from build123d import *

# Parameters (mm, degrees)
P_IDAT_VYSUNUT_M1_DEPTH  = 31
SKICA3_R                 = 3.5
ODEBRAT_VYSUNUT_M1_DEPTH = 4
SKICA4_R                 = 2
ODEBRAT_VYSUNUT_M2_DEPTH = 36.80851854
SKICA5_R                 = 2
ODEBRAT_VYSUNUT_M3_DEPTH = 10


with BuildPart() as part:
    # Skica2 → Přidat vysunutím1 (new body)
    with BuildSketch(Plane.XY):
        with BuildLine():
            Line((15.5, -4.5), (15.5, 4.5))
            Line((15.5, 4.5), (-15.5, 4.5))
            Line((-15.5, 4.5), (-15.5, -4.5))
            Line((-15.5, -4.5), (-4, -4.5))
            ThreePointArc((-4, -4.5), (0, -0.5), (4, -4.5))
            Line((4, -4.5), (15.5, -4.5))
        make_face()
    extrude(amount=P_IDAT_VYSUNUT_M1_DEPTH)

    # Skica3 → Odebrat vysunutím1 (cut)
    with BuildSketch(Plane(origin=(0, 4.5, 0), x_dir=(1, 0, 0), z_dir=(0, 1, 0))):
        with Locations(Location((9.75, -5.75, 0), (0, 0, 270))):
            Circle(SKICA3_R)
        with Locations(Location((9.75, -25.25, 0), (0, 0, 90))):
            Circle(SKICA3_R)
        with Locations(Location((-9.75, -5.75, 0), (0, 0, 90))):
            Circle(SKICA3_R)
        with Locations(Location((-9.75, -25.25, 0), (0, 0, 270))):
            Circle(SKICA3_R)
    extrude(amount=-ODEBRAT_VYSUNUT_M1_DEPTH, mode=Mode.SUBTRACT)

    # Skica4 → Odebrat vysunutím2 (cut, through all)
    with BuildSketch(Plane(origin=(0, 4.5, 0), x_dir=(1, 0, 0), z_dir=(0, 1, 0))):
        with Locations(Location((9.75, -5.75, 0), (0, 0, 270))):
            Circle(SKICA4_R)
        with Locations(Location((-9.75, -5.75, 0), (0, 0, 270))):
            Circle(SKICA4_R)
        with Locations(Location((-9.75, -25.25, 0), (0, 0, 270))):
            Circle(SKICA4_R)
        with Locations(Location((9.75, -25.25, 0), (0, 0, 270))):
            Circle(SKICA4_R)
    extrude(amount=-ODEBRAT_VYSUNUT_M2_DEPTH, mode=Mode.SUBTRACT)

    # Skica5 → Odebrat vysunutím3 (cut)
    with BuildSketch(Plane(origin=(15.5, 0, 0), x_dir=(0, 0, -1), z_dir=(1, 0, 0))):
        with Locations((-15.5, 0)):
            Circle(SKICA5_R)
    extrude(amount=-ODEBRAT_VYSUNUT_M3_DEPTH, mode=Mode.SUBTRACT)


solid = part.part
Work out the finished part from the listing and answer in its coordinate system (mm). A direction names the side the tool comes from. Give positions to 0.01 mm unless a question says otherwise; leave off trailing zeros. Loops run counter-clockwise (first coordinate to the right, second up) from the corner with the lowest first, then second, coordinate; pieces in that order, holes last. Notation, with made-up numbers: (2.5, 33.5) -> (6.5, 33.5) arc R22 cw to (6.5, 49.5) -> close; hole circle Ø1 at (-29, 32). An arc over 180 degrees is marked (long way). Use a Markdown table: item, result. Add a question column.
1. Find the intervals of material crossed by probe 1 along X at (y, z) = (3.15, 25.25); probe 2 along Z at (x, y) = (-9, -0.5); probe 3 along X at (y, z) = (2.25, 3), in increasing order.
2. Section D-D on x = 14.5 is taken. Determine the outline of the cut face in (y, z).
3. Flat-ended cylindrical pins translate along their axes: pin 1 Ø3 at (y, z) = (0, 15.5) entering from +X; pin 2 Ø5 at (x, z) = (0, 9) entering from -Y; pin 3 Ø5.5 at (x, z) = (-9.75, 25.25) entering from +Y. Find the tip coordinate at first contact, or state that the pin passes through.
4. Section B-B on y = -1 is taken. Determine the outline of the cut face in (x, z).
5. Section A-A on x = 9.75 is taken. Determine the outline of the cut face in (y, z).
6. For faces 1 (the flat face through (0, 4.5, 15)), 2 (the cylindrical face through (-11.091, 2.528, 28.483)), 3 (the flat face through (5.5, 0, 16)), determine the directions among +Z, -Z, +X, -X, +Y, -Y from which every point of the face is accessible in a straight line to the end or side of a thin tool.
7. Section C-C on z = 25.25 is taken. Determine the outline of the cut face in (x, y), and give its area (3 significant figures).
8. Determine the mould class of faces 4 (the flat face through (-10, -4.5, 15)), 5 (the cylindrical face through (10.6, -1.2, 17.1)), 6 (the flat face through (-15.5, 0, 15)) for opening direction Y: released by +Y, released by -Y, zero draft, split by the parting line, or undercut.
Results below:
| question | item | result |
|---|---|---|
| 1 | probe 1 | x = -15.5 to -13.25, -6.25 to 6.25, 13.25 to 15.5 |
| 1 | probe 2 | z = 0 to 3.9, 7.6 to 23.4, 27.1 to 31 |
| 1 | probe 3 | x = -15.5 to -11.92, -7.58 to 7.58, 11.92 to 15.5 |
| 2 | outline | (-4.5, 0) -> (4.5, 0) -> (4.5, 31) -> (-4.5, 31) -> close; hole circle Ø4 at (0, 15.5) |
| 3 | pin 1 | stops at x = 5.5 |
| 3 | pin 2 | stops at y = -1.38 |
| 3 | pin 3 | stops at y = 0.5 |
| 4 | outline | (-15.5, 0) -> (-1.94, 0) -> (-1.94, 31) -> (-15.5, 31) -> close; (1.94, 0) -> (15.5, 0) -> (15.5, 13.77) -> (5.5, 13.77) -> (5.5, 17.23) -> (15.5, 17.23) -> (15.5, 31) -> (1.94, 31) -> close; hole circle Ø4 at (-9.75, 5.75); hole circle Ø4 at (-9.75, 25.25); hole circle Ø4 at (9.75, 5.75); hole circle Ø4 at (9.75, 25.25) |
| 5 | outline | (-4.5, 0) -> (4.5, 0) -> (4.5, 2.25) -> (0.5, 2.25) -> (0.5, 3.75) -> (-4.5, 3.75) -> close; (-4.5, 7.75) -> (0.5, 7.75) -> (0.5, 9.25) -> (4.5, 9.25) -> (4.5, 21.75) -> (0.5, 21.75) -> (0.5, 23.25) -> (-4.5, 23.25) -> close; (-4.5, 27.25) -> (0.5, 27.25) -> (0.5, 28.75) -> (4.5, 28.75) -> (4.5, 31) -> (-4.5, 31) -> close; hole circle Ø4 at (0, 15.5) |
| 6 | face 1 | +Z, -Z, +X, -X, +Y |
| 6 | face 2 | +Y |
| 6 | face 3 | +X |
| 7 | outline | (-15.5, -4.5) -> (-11.75, -4.5) -> (-11.75, 0.5) -> (-13.25, 0.5) -> (-13.25, 4.5) -> (-15.5, 4.5) -> close; (-7.75, -4.5) -> (-4, -4.5) arc R4 cw to (4, -4.5) -> (7.75, -4.5) -> (7.75, 0.5) -> (6.25, 0.5) -> (6.25, 4.5) -> (-6.25, 4.5) -> (-6.25, 0.5) -> (-7.75, 0.5) -> close; (11.75, -4.5) -> (15.5, -4.5) -> (15.5, 4.5) -> (13.25, 4.5) -> (13.25, 0.5) -> (11.75, 0.5) -> close |
| 7 | area | 158 mm^2 |
| 8 | face 4 | released by -Y |
| 8 | face 5 | undercut |
| 8 | face 6 | zero draft |
